The figure shows three views and two pictorial views of one solid part (mm, origin at its lowest corner). Answer the questions. Coordinates: 2 decimals unless noted, no trailing zeros. Write each loop counter-clockwise with the first axis right and the second up, starting at its lowest first coordinate (ties: lowest second). Pieces come first, ordered by that corner, then holes.
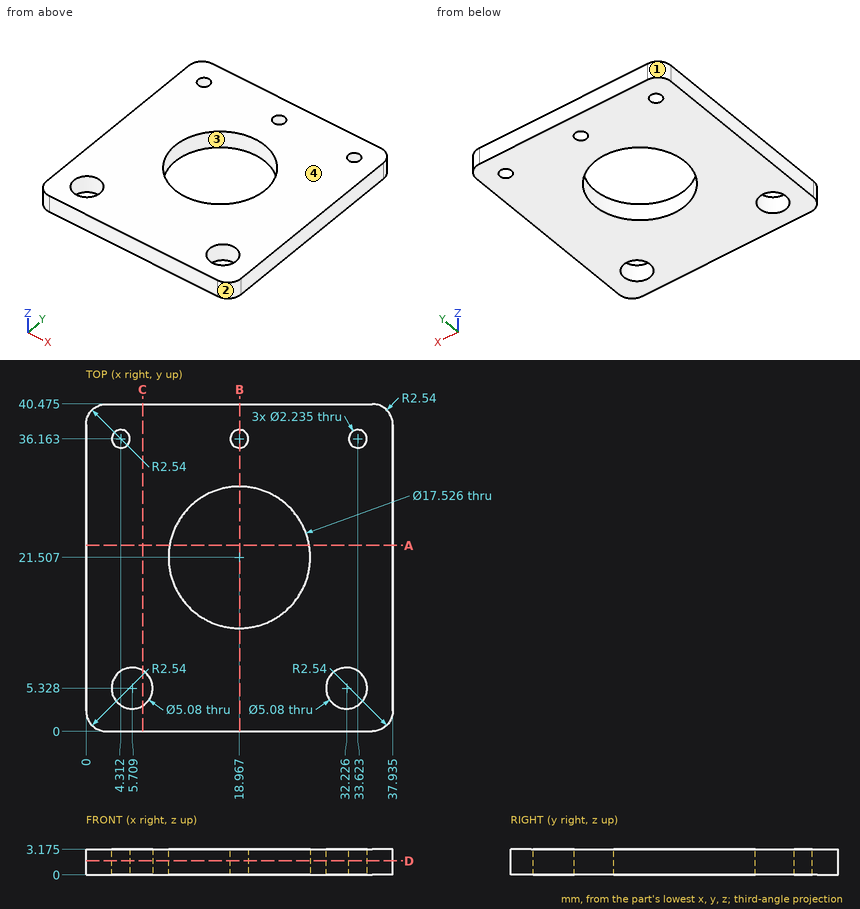
1. For a pull along X with two mould halves and no side action, classify the marked faces 1, 2, 3 and 4 as pulls with the +X half, pulls with the -X half, needs draft (parallel to the pull), parting line crosses it, or undercut.
Results found:
face 1: pulls with the -X half
face 2: pulls with the +X half
face 3: undercut
face 4: needs draft
2. Section C-C on x = 7 is taken. Give the vertices of the cut face in (y, z) (1 decimal), then the cut area to 3 significant figures.
Results found:
outline: (0, 0) - (3.1, 0) - (3.1, 3.2) - (0, 3.2) - close; (7.5, 0) - (40.5, 0) - (40.5, 3.2) - (7.5, 3.2) - close
area: 115 mm2
3. Section A-A on y = 23 is taken. Give the vertices of the cut face in (x, z) (1 decimal).
Results found:
outline: (0, 0) - (10.3, 0) - (10.3, 3.2) - (0, 3.2) - close; (27.6, 0) - (37.9, 0) - (37.9, 3.2) - (27.6, 3.2) - close
4. Find the intervals of material crossed by L1, parallel to X at y = 7.5, z = 3 (1 decimal); L2, parallel to X at y = 3.5, z = 2.3 (1 decimal); L3, parallel to Y at x = 15, z = 2.05 (1 decimal), in increasing order.
Results found:
L1: x = 0 to 4.4, 7 to 30.9, 33.5 to 37.9
L2: x = 0 to 3.9, 7.5 to 30.5, 34 to 37.9
L3: y = 0 to 13.7, 29.3 to 40.5
5. A flat-ended cylindrical pin translates along its axis: P1, Ø16, axis at x = 18.97, y = 21.51, coming from the -Z side. Find the tip coordinate at first contact, or state that the pin passes through.
Results found:
P1: passes through
6. Section B-B on x = 19 is taken. Give the vertices of the cut face in (y, z) (1 decimal).
Results found:
outline: (0, 0) - (12.7, 0) - (12.7, 3.2) - (0, 3.2) - close; (30.3, 0) - (35, 0) - (35, 3.2) - (30.3, 3.2) - close; (37.3, 0) - (40.5, 0) - (40.5, 3.2) - (37.3, 3.2) - close
7. Section D-D on z = 1.75 is taken. Give the vertices of the cut face in (x, y) (1 decimal), then the cut area to 3 significant figures.
Results found:
outline: (0, 2.5) arc R2.5 ccw to (2.5, 0) - (35.4, 0) arc R2.5 ccw to (37.9, 2.5) - (37.9, 37.9) arc R2.5 ccw to (35.4, 40.5) - (2.5, 40.5) arc R2.5 ccw to (0, 37.9) - close; hole circle Ø5.1 at (5.7, 5.3); hole circle Ø2.2 at (4.3, 36.2); hole circle Ø17.5 at (19, 21.5); hole circle Ø2.2 at (19, 36.2); hole circle Ø5.1 at (32.2, 5.3); hole circle Ø2.2 at (33.6, 36.2)
area: 1,240 mm2
